Design review of the part built by this model. Coordinates are the model's own, in mm. A direction names the side the tool comes from. Round coordinates to 2 decimals unless told otherwise and drop trailing zeros. Loops run counter-clockwise (first coordinate to the right, second up) from the corner with the lowest first, then second, coordinate; pieces in that order, holes last. Notation, with made-up numbers: M -28,38 L -4,38 A21 ccw -4,42 Z; hole C 71,4.5 d5. An arc over 180 degrees is marked long. One line per item, written item: value. Start each with the question number.
Item 1: For faces 4 (the flat face through (28.918, 39, 173)), 5 (the flat face through (42, 30.971, 218)), 6 (the flat face through (44, 48.768, 207)), list the 3-axis set-ups (+Z, -Z, +X, -X, +Y, -Y) from which the entire face can be reached by the end or side of a thin tool; tool diameter is ignored.
Item 2: Clearance check with flat-ended pins moving along their axes: pin 1 (3 mm diameter, centred on y = 40, z = 140.5, fed in from -X); pin 2 (22.5 mm diameter, centred on y = 33.5, z = 9, fed in from +X); pin 3 (22.5 mm diameter, centred on y = 40, z = 131, fed in from +X). State where each tip first meets the part, or that it passes through.
Item 3: We need section A-A (x = 56). Write out the cut boundary in (y, z).
Item 4: Mouldability with a two-part tool opening along X and no side actions: class faces 1 (the flat face through (75, 30, 302.613)), 2 (the flat face through (96.35, 38, 312)), 3 (the flat face through (62, 39, 322.86)) as released by +X, released by -X, zero draft, split by the parting line, or undercut.
Item 5: We need section B-B (y = 58). Write out the cut boundary in (x, z).
Item 6: We need section C-C (x = 13). Write out the cut boundary in (y, z).
Item 7: For line 1 along Z through (x, y) = (15, 46.5); line 2 along X through (y, z) = (37, 275.5); line 3 along Y through (x, z) = (40, 133), list the stretches that pass through material, from the lowest coordinate up.
Item 8: We need section D-D (z = 60). Write out the cut boundary in (x, y).
from build123d import *

# Parameters (mm, degrees)
F0_W        = 76.344192028
F0_H        = 75.5144134164
F1_DEPTH    = 25.4
F2_W        = 17.4319148064
F2_H        = 20.3372240067
F3_DEPTH    = 300
F4_W        = 20.3372240067
F4_H        = 22.7871290684
F5_DEPTH    = 50
F6_F1_R     = 5.08
F6_F2_R     = 5.08
F7_T        = 2.54
F7_T3_DEPTH = 10.16
F7_T5_DEPTH = 25.4172240067
F7_T7_DEPTH = 10.16
F8_R        = 5.08


# Not quite as in the source:
# - a shell that OpenCascade refuses in one call is made with other operations: the cavity is built on its own and cut out


with BuildPart() as f1:
    # F0 (on Top) → F1 (new body)
    with BuildSketch(Plane.XY):
        with Locations((38.172096014, 37.7572067082)):
            Rectangle(F0_W, F0_H)
    extrude(amount=F1_DEPTH)

    # F2 (on face) → F3 (join)
    with BuildSketch(Plane.XY.offset(25.4)):
        with Locations((37.6336574554, 38.5992005467)):
            Rectangle(F2_W, F2_H)
    extrude(amount=F3_DEPTH)

    # F4 (on face) → F5 (join)
    with BuildSketch(Plane.YZ.offset(46.3496148586)):
        with Locations((38.5992005467, 314.0064354658)):
            Rectangle(F4_W, F4_H)
    extrude(amount=F5_DEPTH)

    # F6: fillet of radius 5.08 on 7 edges, made by hand

    # F6_f1
    f6_f1_edges = [f1.edges().sort_by_distance(p)[0] for p in [
        (28.9177000523, 48.7678125501, 175.4),
        (28.9177000523, 28.4305885434, 175.4),
        (28.9177000523, 38.5992005467, 325.4),
        (62.6336574554, 48.7678125501, 325.4),
        (62.6336574554, 28.4305885434, 325.4),
        (96.3496148586, 38.5992005467, 325.4),
    ]]
    fillet(f6_f1_edges, radius=F6_F1_R)

    # F6_f2
    f6_f2_edges = [f1.edges().sort_by_distance(p)[0] for p in [
        (28.9177000523, 38.5992005467, 25.4),
        (30.4055976038, 47.2799149985, 25.4),
        (30.4055976038, 29.918486095, 25.4),
    ]]
    fillet(f6_f2_edges, radius=F6_F2_R)

    # F7: shell of thickness 2.54, made by hand


with BuildPart() as f7_core1:
    # F7_t2: copy of F1
    add(f1.part)

    # the walls: a layer under each face that stays
    f7_faces = [f7_core1.faces().sort_by_distance(p)[0] for p in [
        (12.7240320047, 12.5857355694, 25.4),
        (46.3496148586, 38.5992005467, 164.0064354658),
        (40.1736574554, 50.2557101016, 26.8878975516),
        (29.3534951554, 48.3320174469, 26.8878975516),
        (40.1736574554, 26.9426909918, 26.8878975516),
        (27.4298025007, 38.5992005467, 26.8878975516),
        (29.3534951554, 28.8663836466, 26.8878975516),
        (0, 37.7572067082, 12.7),
        (38.172096014, 75.5144134164, 12.7),
        (38.172096014, 0, 12.7),
        (76.344192028, 37.7572067082, 12.7),
        (44.3896858533, 48.7678125501, 272.0133333333),
        (44.3896858533, 28.4305885434, 272.0133333333),
        (30.4055976038, 47.2799149985, 175.4),
        (28.9177000523, 38.5992005467, 175.4),
        (30.4055976038, 29.918486095, 175.4),
        (38.172096014, 37.7572067082, 0),
        (65.1736574554, 47.2799149985, 323.9121024484),
        (96.3496148586, 38.5992005467, 311.4664354658),
        (65.1736574554, 29.918486095, 323.9121024484),
        (31.4577000523, 46.2278125501, 323.9121024484),
        (30.4055976038, 38.5992005467, 323.9121024484),
        (31.4577000523, 30.9705885434, 323.9121024484),
        (62.6336574554, 38.5992005467, 325.4),
        (94.8617173071, 38.5992005467, 323.9121024484),
    ]]
    thicken(f7_faces, amount=-F7_T, mode=Mode.SUBTRACT)

    # F7_s4 → F7_t3 (cut)
    with BuildSketch(Plane.XZ.offset(-56.3878125501)):
        Polygon((46.3750148586, 25.4254), (46.3496148586, 22.86), (43.8096148586, 22.86), (43.8096148586, 25.4), align=None)
    extrude(amount=F7_T3_DEPTH, mode=Mode.SUBTRACT)

    # F7_s6 → F7_t5 (cut)
    with BuildSketch(Plane.XZ.offset(-51.3078125501)):
        Polygon((46.3750148586, 25.4254), (46.3496148586, 22.86), (43.8096148586, 22.86), (43.8096148586, 25.4), align=None)
    extrude(amount=F7_T5_DEPTH, mode=Mode.SUBTRACT)

    # F7_s8 → F7_t7 (cut)
    with BuildSketch(Plane.XZ.offset(-30.9705885434)):
        Polygon((46.3750148586, 25.4254), (46.3496148586, 22.86), (43.8096148586, 22.86), (43.8096148586, 25.4), align=None)
    extrude(amount=F7_T7_DEPTH, mode=Mode.SUBTRACT)


with BuildPart() as f1_1:
    add(f1.part)

    # what is left inside the walls is the cavity
    f7_cavity = [f7_core1.part.solids().sort_by_distance(p)[0] for p in [
        (38.172096, 26.018138, 2.5654),
    ]]
    add(f7_cavity, mode=Mode.SUBTRACT)

    # F8
    f8_edges = [f1_1.edges().sort_by_distance(p)[0] for p in [
        (46.349615, 38.599201, 25.4),
        (40.173657, 23.350589, 25.4),
        (26.813495, 26.326384, 25.4),
        (23.8377, 38.599201, 25.4),
        (26.813495, 50.872017, 25.4),
        (40.173657, 53.847813, 25.4),
        (0, 37.757207, 25.4),
        (38.172096, 0, 25.4),
        (76.344192, 37.757207, 25.4),
        (38.172096, 75.514413, 25.4),
    ]]
    fillet(f8_edges, radius=F8_R)


solid = f1_1.part
A:
1. face 4: +Z, -X, +Y, -Y
1. face 5: none
1. face 6: +Z, +X, -X, +Y
2. pin 1: x = 28.92
2. pin 2: x = 76.34
2. pin 3: x = 46.35
3. outline: M 0,0 L 75.51,0 L 75.51,20.32 A5.08 ccw 70.43,25.4 L 5.08,25.4 A5.08 ccw 0,20.32 Z; M 28.43,302.61 L 30.97,302.61 L 30.97,320.32 A2.54 cw 33.51,322.86 L 43.69,322.86 A2.54 cw 46.23,320.32 L 46.23,302.61 L 48.77,302.61 L 48.77,320.32 A5.08 ccw 43.69,325.4 L 33.51,325.4 A5.08 ccw 28.43,320.32 Z; hole M 2.54,2.54 L 72.97,2.54 L 72.97,22.86 L 2.54,22.86 Z
4. face 1: zero draft
4. face 2: released by +X
4. face 3: undercut
5. outline: M 0,0 L 76.34,0 L 76.34,20.32 A5.08 ccw 71.26,25.4 L 5.08,25.4 A5.08 ccw 0,20.32 Z; hole M 2.54,2.54 L 73.8,2.54 L 73.8,22.86 L 2.54,22.86 Z
6. outline: M 0,0 L 75.51,0 L 75.51,20.32 A5.08 ccw 70.43,25.4 L 5.08,25.4 A5.08 ccw 0,20.32 Z; hole M 2.54,2.54 L 72.97,2.54 L 72.97,22.86 L 2.54,22.86 Z
7. line 1: 0 to 2.54, 22.86 to 25.4
7. line 2: 28.92 to 31.46, 43.81 to 46.35
7. line 3: 28.43 to 30.97, 46.23 to 48.77
8. outline: M 28.92,33.51 A5.08 ccw 34,28.43 L 46.35,28.43 L 46.35,48.77 L 34,48.77 A5.08 ccw 28.92,43.69 Z; hole M 31.46,33.51 A2.54 ccw 34,30.97 L 43.81,30.97 L 43.81,46.23 L 34,46.23 A2.54 ccw 31.46,43.69 Z
